Can you work these out from the model? Positions are in its coordinate system, mm. Face numbers are marked on the shaded views. A direction names the side the tool comes from. Coordinates: 2 decimals unless noted, no trailing zeros. Loops run counter-clockwise (first coordinate to the right, second up) from the corner with the lowest first, then second, coordinate; pieces in that order, holes last. Notation, with made-up numbers: M 33,68 L 73,68 A23 cw 73,77 Z; hole C -13,-40 d2. An arc over 180 degrees is marked long. Return JSON: item names as keys, results as strings. Group by question number.
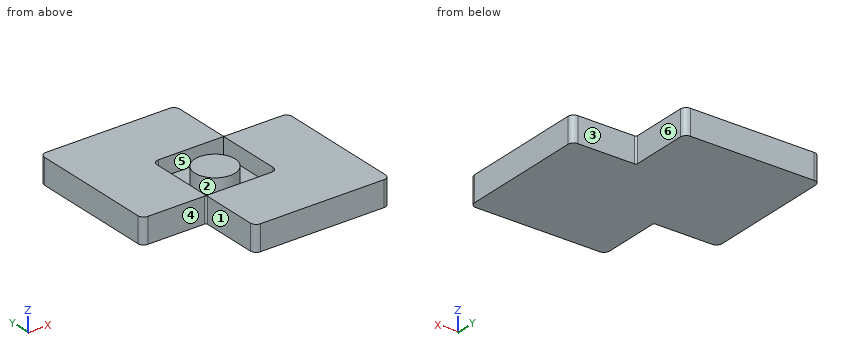
```python
from build123d import *

# Parameters (mm, degrees)
F1_DEPTH = 1.5
F2_R     = 0.1
F3_DEPTH = 1


with BuildPart() as f1:
    # F0 (on Top) → F1 (new body)
    with BuildSketch(Plane.XY):
        with BuildLine():
            Line((1.762745, 5.894785), (-5.552315, 5.894785))
            ThreePointArc((-5.552315, 5.894785), (-5.794478, 5.794478), (-5.894785, 5.552315))
            Line((-5.894785, 5.552315), (-5.894785, -1.762745))
            ThreePointArc((-5.894785, -1.762745), (-5.794478, -2.004908), (-5.552315, -2.105215))
            Line((-5.552315, -2.105215), (-2.105215, -2.105215))
            Line((-2.105215, -2.105215), (-2.105215, 1.762745))
            ThreePointArc((-2.105215, 1.762745), (-2.004908, 2.004908), (-1.762745, 2.105215))
            Line((-1.762745, 2.105215), (2.105215, 2.105215))
            Line((2.105215, 2.105215), (2.105215, 5.552315))
            ThreePointArc((2.105215, 5.552315), (2.004908, 5.794478), (1.762745, 5.894785))
        make_face()
        with BuildLine():
            Line((2.105215, -1.762745), (2.105215, 2.105215))
            Line((2.105215, 2.105215), (-1.762745, 2.105215))
            ThreePointArc((-1.762745, 2.105215), (-2.004908, 2.004908), (-2.105215, 1.762745))
            Line((-2.105215, 1.762745), (-2.105215, -2.105215))
            Line((-2.105215, -2.105215), (1.762745, -2.105215))
            ThreePointArc((1.762745, -2.105215), (2.004908, -2.004908), (2.105215, -1.762745))
        make_face()
        with BuildLine():
            ThreePointArc((0.840188, 0.840188), (0.840188, -0.840188), (-0.840188, -0.840188))
            ThreePointArc((-0.840188, -0.840188), (-0.840188, 0.840188), (0.840188, 0.840188))
        make_face(mode=Mode.SUBTRACT)
        with BuildLine():
            ThreePointArc((0.840188, 0.840188), (-0.840188, 0.840188), (-0.840188, -0.840188))
            ThreePointArc((-0.840188, -0.840188), (0.840188, -0.840188), (0.840188, 0.840188))
        make_face()
        with BuildLine():
            Line((5.552315, 2.105215), (2.105215, 2.105215))
            Line((2.105215, 2.105215), (2.105215, -1.762745))
            ThreePointArc((2.105215, -1.762745), (2.004908, -2.004908), (1.762745, -2.105215))
            Line((1.762745, -2.105215), (-2.105215, -2.105215))
            Line((-2.105215, -2.105215), (-2.105215, -5.552315))
            ThreePointArc((-2.105215, -5.552315), (-2.004908, -5.794478), (-1.762745, -5.894785))
            Line((-1.762745, -5.894785), (5.552315, -5.894785))
            ThreePointArc((5.552315, -5.894785), (5.794478, -5.794478), (5.894785, -5.552315))
            Line((5.894785, -5.552315), (5.894785, 1.762745))
            ThreePointArc((5.894785, 1.762745), (5.794478, 2.004908), (5.552315, 2.105215))
        make_face()
    extrude(amount=-F1_DEPTH)

    # F2
    f2_edges = [f1.edges().sort_by_distance(p)[0] for p in [
        (-2.105215, -2.105215, -0.75),
        (2.105215, 2.105215, -0.75),
    ]]
    fillet(f2_edges, radius=F2_R)

    # F0 (on Top) → F3 (cut)
    with BuildSketch(Plane.XY):
        with BuildLine():
            Line((2.105215, -1.762745), (2.105215, 2.105215))
            Line((2.105215, 2.105215), (-1.762745, 2.105215))
            ThreePointArc((-1.762745, 2.105215), (-2.004908, 2.004908), (-2.105215, 1.762745))
            Line((-2.105215, 1.762745), (-2.105215, -2.105215))
            Line((-2.105215, -2.105215), (1.762745, -2.105215))
            ThreePointArc((1.762745, -2.105215), (2.004908, -2.004908), (2.105215, -1.762745))
        make_face()
        with BuildLine():
            ThreePointArc((0.840188, 0.840188), (0.840188, -0.840188), (-0.840188, -0.840188))
            ThreePointArc((-0.840188, -0.840188), (-0.840188, 0.840188), (0.840188, 0.840188))
        make_face(mode=Mode.SUBTRACT)
    extrude(amount=-F3_DEPTH, mode=Mode.SUBTRACT)


solid = f1.part
```
1) Suppose I cut it at A-A, the plane z = -0.35. List the corners of the cut face in (x, y) for me, then the cut area to 3 significant figures.
2) Suppose I cut it at B-B, the plane x = 0. List the corners of the cut face in (y, z) for me, then the cut area to 3 significant figures.
3) Suppose I cut it at D-D, the plane x = -2.5. List the corners of the cut face in (y, z) for me, then the cut area to 3 significant figures.
4) If we mould it in two halves opening along Y, with no side actions, what happens to the marked faces 1, 2 and 3? For each: +Y half, -Y half, draft (parallel to the pull), parting line (faces both ways), or undercut.
5) If I drill on line 1 (Y direction, x = 0, z = -0.8); line 2 (X direction, y = -1, z = -0.65); line 3 (X direction, y = -5, z = -0.05), over which ranges is the centre line in solid material (lowest first)? Write a range as from..to.
6) For the marked faces 4, 5 and 6, which set-ups out of +Z, -Z, +X, -X, +Y, -Y let a thin tool reach every point of the face, with its end or its side?
7) For pin 1 (0.8 mm diameter, centred on x = -3.5, z = -0.5, fed in from -Y); pin 2 (2 mm diameter, centred on x = -0.5, y = 0.5, fed in from +Z), each with a flat end and sliding along its axis, tell me the tip position at first contact or that it passes through.
Returned:
{
 "1": {"outline": "M -5.89,-1.76 A0.34 ccw -5.55,-2.11 L -2.21,-2.11 A0.1 cw -2.11,-2.21 L -2.11,-5.55 A0.34 ccw -1.76,-5.89 L 5.55,-5.89 A0.34 ccw 5.89,-5.55 L 5.89,1.76 A0.34 ccw 5.55,2.11 L 2.21,2.11 A0.1 cw 2.11,2.21 L 2.11,5.55 A0.34 ccw 1.76,5.89 L -5.55,5.89 A0.34 ccw -5.89,5.55 Z; C 0,0 d2.38; hole M -2.11,-2.11 L 1.76,-2.11 A0.34 ccw 2.11,-1.76 L 2.11,2.11 L -1.76,2.11 A0.34 ccw -2.11,1.76 Z", "area": "96.9 mm²"},
 "2": {"outline": "M -5.89,-1.5 L 5.89,-1.5 L 5.89,0 L 2.11,0 L 2.11,-1 L 1.19,-1 L 1.19,0 L -1.19,0 L -1.19,-1 L -2.11,-1 L -2.11,0 L -5.89,0 Z", "area": "15.9 mm²"},
 "3": {"outline": "M -2.11,-1.5 L 5.89,-1.5 L 5.89,0 L -2.11,0 Z", "area": "12.0 mm²"},
 "4": {"face 1": "draft", "face 2": "undercut", "face 3": "+Y half"},
 "5": {"line 1": "y = -5.89..-2.11, -1.19..1.19, 2.11..5.89", "line 2": "x = -5.89..-2.11, -0.64..0.64, 2.11..5.89", "line 3": "x = -2.11..5.89"},
 "6": {"face 4": "+Z, -Z, -X, -Y", "face 5": "+Z", "face 6": "+Z, -Z, +X, +Y"},
 "7": {"pin 1": "stops at y = -2.11", "pin 2": "stops at z = 0"}
}
